For this review, take the finished solid that the model builds, in its own axes (mm). A direction names the side the tool comes from. Coordinates: 2 decimals unless noted, no trailing zeros. Loops run counter-clockwise (first coordinate to the right, second up) from the corner with the lowest first, then second, coordinate; pieces in that order, holes last. Notation, with made-up numbers: (41, 27.5) - (86, 27.5) arc R24 cw to (86, 45.5) - close; hole circle Ø6 at (69, 27). An arc over 180 degrees is marked (long way). Use one line per item in the form item = value. Start each with the question number.
1. To check wall thickness, follow probe 1 along Y at (x, z) = (28, 18.75); probe 2 along Y at (x, z) = (26, 12). State the ranges of each line that lie inside material, in increasing order.
2. Add section C-C on z = 14. Give the boundary of the cut face in (x, y).
3. Add section A-A on z = 19. Give the boundary of the cut face in (x, y), and give its area (3 significant figures).
4. Draft analysis for pull direction Y (two halves, no side actions). For faces 1 (the face through (-1, -40, 12)), 2 (the face through (-1, -15, 25)), 3 (the face through (0.56, 19.289, 11.804)), state which applies: +Y half, -Y half, draft (parallel to the pull), parting line (faces both ways), or undercut.
5. Add section D-D on y = 12. Give the boundary of the cut face in (x, z).
6. Machinability: for faces 4 (the face through (-1, 21, 21)), 5 (the face through (-1, 1, 0)), which of the approach directions +Z, -Z, +X, -X, +Y, -Y give a long, thin tool a straight path to every point of the face, cutting with its end or side? Answer none if there is none.
```python
from build123d import *

# Parameters (mm, degrees)
F0_W     = 80
F0_H     = 80
F1_DEPTH = 25
F2_W     = 80
F2_H     = 12
F3_DEPTH = 15
F4_R     = 5.99999


# Not quite as in the source:
# - a fillet or chamfer is up to 0.001 mm smaller than in the source, because OpenCascade refuses the exact size


with BuildPart() as f1:
    # F0 (on Top) → F1 (new body)
    with BuildSketch(Plane.XY):
        Rectangle(F0_W, F0_H)
    extrude(amount=F1_DEPTH)

    # F2 (on face) → F3 (cut)
    with BuildSketch(Plane.XY.offset(25)):
        with Locations((0, 15)):
            Rectangle(F2_W, F2_H)
    extrude(amount=-F3_DEPTH, mode=Mode.SUBTRACT)

    # F4 (radius 6 in the source; OpenCascade refuses exactly that, so slightly less here)
    f4_edges = [f1.edges().sort_by_distance(p)[0] for p in [
        (0, 9, 10),
        (0, 21, 10),
    ]]
    fillet(f4_edges, radius=F4_R)


solid = f1.part
```
Conclusion:
q1.probe_1 = -40 to 9, 21 to 40
q1.probe_2 = -40 to 10.53, 19.47 to 40
q2.outline = (-40, -40) - (40, -40) - (40, 9.34) - (-40, 9.34) - close; (-40, 20.66) - (40, 20.66) - (40, 40) - (-40, 40) - close
q3.outline = (-40, -40) - (40, -40) - (40, 9) - (-40, 9) - close; (-40, 21) - (40, 21) - (40, 40) - (-40, 40) - close
q3.area = 5,440 mm^2
q4.face_1 = -Y half
q4.face_2 = draft
q4.face_3 = undercut
q5.outline = (-40, 0) - (40, 0) - (40, 10.8) - (-40, 10.8) - close
q6.face_4 = +Z, +X, -X
q6.face_5 = -Z, +X, -X, +Y, -Y
